CAD build for the part. Positions are in the model's coordinates, mm. Face numbers are marked on the shaded views. A direction names the side the tool comes from. Give positions to 0.01 mm unless a question says otherwise; leave off trailing zeros. Order: outer loops, then holes, each group sorted by start corner. A loop starts at its lowest first (then second) coordinate and runs counter-clockwise, first axis right, second up. Notation, with made-up numbers: (69, 60.5) -> (120, 60.5) arc R20 cw to (120, 94.5) -> close; hole circle Ø5 at (61, -33.5). An arc over 180 degrees is marked (long way). Answer as CSV lines item,"result".
```python
from build123d import *

# Parameters (mm, degrees)
SKETCH1_R           = 5
BOSS_EXTRUDE1_DEPTH = 10
BOSS_EXTRUDE2_DEPTH = 10
SKETCH3_W           = 20
SKETCH3_H           = 20
SKETCH3_W_2         = 15
SKETCH3_H_2         = 15
BOSS_EXTRUDE3_DEPTH = 21
SKETCH4_W           = 50
SKETCH4_H           = 50
BOSS_EXTRUDE4_DEPTH = 3
SKETCH5_R           = 10
BOSS_EXTRUDE5_DEPTH = 100
BOSS_EXTRUDE6_DEPTH = 5


with BuildPart() as part:
    # Sketch1 → Boss-Extrude1 (new body)
    with BuildSketch(Plane(origin=(0, 0, 0), x_dir=(1, 0, 0), z_dir=(0, 1, 0))):
        with BuildLine():
            Line((0, 0), (30.876052193, 0))
            Line((30.876052193, 0), (30.876052193, -11.362717468))
            ThreePointArc((30.876052193, -11.362717468), (46.762190972, -21.786248919), (50, -3.063642105))
            Line((50, -3.063642105), (50, 0))
            Line((50, 0), (50, 50))
            Line((50, 50), (0, 50))
            Line((0, 50), (0, 0))
        make_face()
        with Locations(Location((42.238769661, -11.362717468, 0), (0, 0, 270))):
            Circle(SKETCH1_R, mode=Mode.SUBTRACT)
        with BuildLine():
            Line((9.874654059, 47.191553979), (24.296746366, 33.290272916))
            ThreePointArc((24.296746366, 33.290272916), (24.424993645, 26.799159409), (17.934255558, 26.653142217))
            Line((17.934255558, 26.653142217), (3.436266044, 40.475249935))
            ThreePointArc((3.436266044, 40.475249935), (3.288101967, 47.061421086), (9.874654059, 47.191553979))
        make_face(mode=Mode.SUBTRACT)
    extrude(amount=BOSS_EXTRUDE1_DEPTH)

    # Sketch2 → Boss-Extrude2 (add)
    with BuildSketch(Plane.XZ):
        Polygon((45, -5), (35, -5), (35, 0), (50, 0), (50, -15), (45, -15), align=None)
    extrude(amount=BOSS_EXTRUDE2_DEPTH)

    # Sketch3 → Boss-Extrude3 (add)
    with BuildSketch(Plane(origin=(0, 10, 0), x_dir=(1, 0, 0), z_dir=(0, 1, 0))):
        with Locations((10, 10)):
            Rectangle(SKETCH3_W, SKETCH3_H)
        with Locations((42.5, 42.5)):
            Rectangle(SKETCH3_W_2, SKETCH3_H_2)
    extrude(amount=BOSS_EXTRUDE3_DEPTH)

    # Sketch4 → Boss-Extrude4 (add)
    with BuildSketch(Plane(origin=(0, 31, 0), x_dir=(1, 0, 0), z_dir=(0, 1, 0))):
        with Locations((25, 25)):
            Rectangle(SKETCH4_W, SKETCH4_H)
    extrude(amount=BOSS_EXTRUDE4_DEPTH)

    # Sketch5 → Boss-Extrude5 (add)
    with BuildSketch(Plane(origin=(0, 34, 0), x_dir=(1, 0, 0), z_dir=(0, 1, 0))):
        with Locations(Location((25, 25, 0), (0, 0, 270))):
            Circle(SKETCH5_R)
    extrude(amount=BOSS_EXTRUDE5_DEPTH)

    # Sketch6 → Boss-Extrude6 (add)
    with BuildSketch(Plane(origin=(0, 134, 0), x_dir=(1, 0, 0), z_dir=(0, 1, 0))):
        with BuildLine():
            Line((35, 25), (35, -25))
            Line((35, -25), (15, -25))
            Line((15, -25), (15, 25))
            ThreePointArc((15, 25), (25, 35), (35, 25))
        make_face()
    extrude(amount=BOSS_EXTRUDE6_DEPTH)


solid = part.part
```
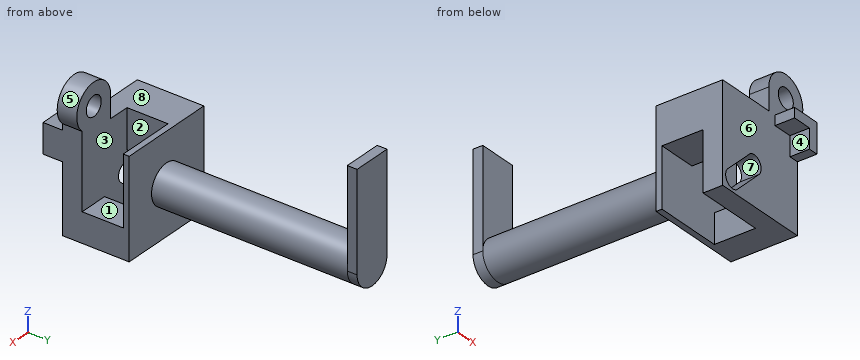
1) Band-saw the part on D-D, the plane y = 101. Write the cut outline in (x, z), then the cut area to 3 significant figures.
Data:
outline,"circle Ø20 at (25, -25)"
area,"314 mm2"
2) Band-saw the part on A-A, the plane y = 20.5. Write the cut outline in (x, z), then the cut area to 3 significant figures.
Data:
outline,"(0, -20) -> (20, -20) -> (20, 0) -> (0, 0) -> close; (35, -50) -> (50, -50) -> (50, -35) -> (35, -35) -> close"
area,"625 mm2"
3) Wall check: line 1 along Y through (x, z) = (41.5, -31); line 2 along Y through (x, z) = (21, -24); line 3 along Y through (x, z) = (49, 15.5). Give the ranges that are in metal, low to high. Write a range as [from, to].
Data:
line 1,"y = [0, 10], [31, 34]"
line 2,"y = [0, 10], [31, 139]"
line 3,"y = [0, 10]"
4) Band-saw the part on C-C, the plane x = 33.5. Write the cut outline in (y, z).
Data:
outline,"(0, -50) -> (10, -50) -> (10, 18.63) -> (0, 18.63) -> close; (31, -50) -> (34, -50) -> (34, -30.27) -> (139, -30.27) -> (139, 25) -> (134, 25) -> (134, -19.73) -> (34, -19.73) -> (34, 0) -> (31, 0) -> close"
5) Pull direction Z, two halves, no side cores. Call the marked faces 5, 6, 7 and 8: pulls with the +Z half, pulls with the -Z half, needs draft (parallel to the pull), parting line crosses it, or undercut.
Data:
face 5,"parting line crosses it"
face 6,"needs draft"
face 7,"undercut"
face 8,"pulls with the +Z half"
6) Which spindle directions (+Z, -Z, +X, -X, +Y, -Y) get a long thin tool onto all of the face, cutting with end or side? Do the marked faces 1, 2, 3 and 4. Say none if no direction does.
Data:
face 1,"+Z, +X, -X"
face 2,"+Z, -Z, +X"
face 3,"none"
face 4,"-Z, -X, -Y"
7) Band-saw the part on B-B, the plane z = -22. Write the cut outline in (x, y).
Data:
outline,"(0, 0) -> (50, 0) -> (50, 10) -> (0, 10) -> close; (0, 31) -> (50, 31) -> (50, 34) -> (34.54, 34) -> (34.54, 134) -> (35, 134) -> (35, 139) -> (15, 139) -> (15, 134) -> (15.46, 134) -> (15.46, 34) -> (0, 34) -> close"
8) Pin check, flat tips, straight feed: P1, Ø6, axis at x = 41.5, z = -37, coming from the -Y side; P2, Ø8, axis at y = 97.5, z = -35.5, coming from the +X side; P3, Ø4, axis at y = -2.5, z = -3.5, coming from the -X side. Stop position of each tip, or through.
Data:
P1,"stops at y = 0"
P2,"stops at x = 32.6"
P3,"stops at x = 35"
